Answer from the drawing. Dimensions are ordinates in mm from the lowest x, y and z of the part. Round coordinates to 2 decimals unless told otherwise and drop trailing zeros. Order: outer loops, then holes, each group sorted by start corner. A loop starts at its lowest first (then second) coordinate and runs counter-clockwise, first axis right, second up. Notation, with made-up numbers: (2.25, 14.25) -> (48.25, 14.25) arc R15 cw to (48.25, 25.25) -> close; hole circle Ø9 at (-18.5, 15.25). An arc over 180 degrees is marked (long way). Use a Markdown table: item, result. Add a question column.
1. Section A-A, the plane z = 25 is taken. Give the vertices of the cut face in (x, y), then the cut area to 3 significant figures.
2. Section C-C, the plane x = 70 is taken. Give the vertices of the cut face in (y, z), then the cut area to 3 significant figures.
3. Section D-D, the plane x = 120 is taken. Give the vertices of the cut face in (y, z).
4. Given pin 1 (5.5 mm diameter, centred on x = 120, y = 15, fed in from +Z), flat-ended and moving along its own axis, determine where the tip first touches the part or whether it passes through.
5. Section B-B, the plane y = 15 is taken. Give the vertices of the cut face in (x, z), then the cut area to 3 significant figures.
6. Consider L1, parallel to X at y = 22.75, z = 25; L2, parallel to Y at x = 45, z = 33; L3, parallel to Y at x = 41, z = 50.5. Determine where each line is inside the solid, lowest interval first. Write a range as [from, to].
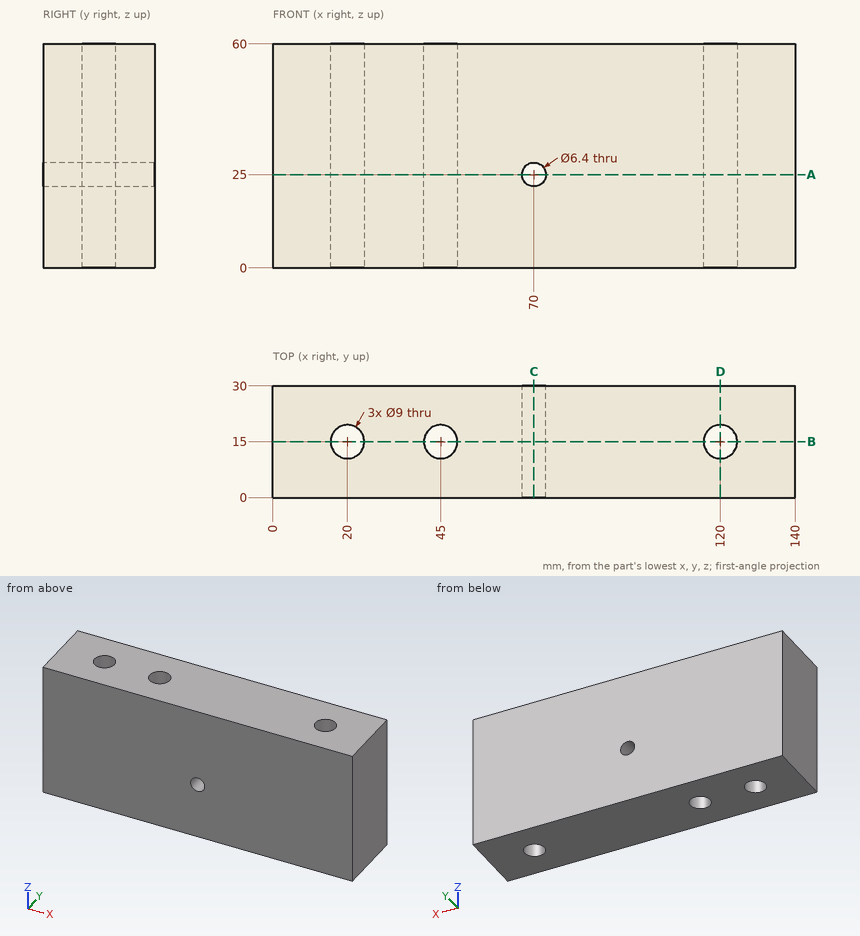
Verdict:
| question | item | result |
|---|---|---|
| 1 | outline | (0, 0) -> (66.8, 0) -> (66.8, 30) -> (0, 30) -> close; (73.2, 0) -> (140, 0) -> (140, 30) -> (73.2, 30) -> close; hole circle Ø9 at (20, 15); hole circle Ø9 at (45, 15); hole circle Ø9 at (120, 15) |
| 1 | area | 3,820 mm2 |
| 2 | outline | (0, 0) -> (30, 0) -> (30, 21.8) -> (0, 21.8) -> close; (0, 28.2) -> (30, 28.2) -> (30, 60) -> (0, 60) -> close |
| 2 | area | 1,610 mm2 |
| 3 | outline | (0, 0) -> (10.5, 0) -> (10.5, 60) -> (0, 60) -> close; (19.5, 0) -> (30, 0) -> (30, 60) -> (19.5, 60) -> close |
| 4 | pin 1 | passes through |
| 5 | outline | (0, 0) -> (15.5, 0) -> (15.5, 60) -> (0, 60) -> close; (24.5, 0) -> (40.5, 0) -> (40.5, 60) -> (24.5, 60) -> close; (49.5, 0) -> (115.5, 0) -> (115.5, 60) -> (49.5, 60) -> close; (124.5, 0) -> (140, 0) -> (140, 60) -> (124.5, 60) -> close; hole circle Ø6.4 at (70, 25) |
| 5 | area | 6,750 mm2 |
| 6 | L1 | x = [0, 66.8], [73.2, 140] |
| 6 | L2 | y = [0, 10.5], [19.5, 30] |
| 6 | L3 | y = [0, 12.94], [17.06, 30] |
